Input: part model. Units: mm. Frame: model coordinates. A direction names the side the tool comes from. Give positions to 0.01 mm unless a question says otherwise; leave off trailing zeros. Loops run counter-clockwise (first coordinate to the right, second up) from the corner with the lowest first, then second, coordinate; pieces in that order, holes last. Notation, with made-up numbers: (-12.5, 3) -> (3.5, 3) arc R18 cw to (3.5, 25) -> close; hole circle Ø3 at (86, 36). An arc over 180 degrees is marked (long way). Answer in a Markdown table with one row per item. Add a question column.
```python
from build123d import *

# Parameters (mm, degrees)
SKETCH_2_R               = 101.541015805
CUT_EXTRUDE_1_DEPTH      = 92
SKETCH_4_R               = 60
SKETCH_4_R_2             = 39
EXTRUDE_1_DEPTH          = 1.5
SKETCH_5_W               = 2
SKETCH_5_H               = 2
CUT_EXTRUDE_2_DEPTH      = 94.808315196
CUT_EXTRUDE_2_DEPTH_BACK = 94.808315196
SKETCH_6_OUTSIDE_W       = 156.966
SKETCH_6_OUTSIDE_H       = 156.966
SKETCH_6_OUTSIDE_R       = 52.5
CUT_EXTRUDE_3_DEPTH      = 84.634622017
CUT_EXTRUDE_3_DEPTH_BACK = 84.634622017
SKETCH_7_OUTSIDE_W       = 137.864
SKETCH_7_OUTSIDE_H       = 137.864
SKETCH_7_OUTSIDE_R       = 50.5


with BuildPart() as part:
    # 草图1 → 旋转1 (revolve)
    with BuildSketch(Plane(origin=(0, 0, 0), x_dir=(0, 0, -1), z_dir=(1, 0, 0))):
        with BuildLine():
            Line((-40, 0), (40, 0))
            ThreePointArc((40, 0), (0, 40), (-40, 0))
        make_face()
    revolve(axis=Axis((0, 0, 40), (0, 0, -1)))

    # 草图2 → 切除-拉伸1 (cut)
    with BuildSketch(Plane.XY):
        with Locations((-18.762206379, 13.237665106)):
            Circle(SKETCH_2_R)
    extrude(amount=-CUT_EXTRUDE_1_DEPTH, mode=Mode.SUBTRACT)

    # 草图3 → 切除-旋转1 (revolve, cut)
    with BuildSketch(Plane(origin=(0, 0, 0), x_dir=(1, 0, 0), z_dir=(0, 1, 0))):
        with BuildLine():
            Line((0, 38.5), (0, -38.5))
            ThreePointArc((0, -38.5), (38.5, 0), (0, 38.5))
        make_face()
    revolve(axis=Axis((0, 0, -38.5), (0, 0, 1)), mode=Mode.SUBTRACT)

    # 草图4 → 凸台-拉伸1 (add)
    with BuildSketch(Plane(origin=(0, 0, 0), x_dir=(-1, 0, 0), z_dir=(0, 0, -1))):
        Circle(SKETCH_4_R)
        Circle(SKETCH_4_R_2, mode=Mode.SUBTRACT)
    extrude(amount=-EXTRUDE_1_DEPTH)

    # 草图5 → 旋转2 (revolve)
    with BuildSketch(Plane(origin=(0, 0, 0), x_dir=(1, 0, 0), z_dir=(0, 1, 0)), mode=Mode.PRIVATE) as revolve_2_sk:
        with Locations((-44, 1)):
            Rectangle(SKETCH_5_W, SKETCH_5_H)
    revolve(revolve_2_sk.sketch.rotate(Axis((0, 0, -24.660694069), (0, 0, 1)), 270), axis=Axis((0, 0, -24.660694069), (0, 0, 1)))

    # 草图6 outside → 切除-拉伸2 (cut, two sides: drawn at the far end of the back side and taken through both)
    with BuildSketch(Plane(origin=(0, 0, 0), x_dir=(-1, 0, 0), z_dir=(0, 0, -1)).offset(-CUT_EXTRUDE_2_DEPTH_BACK)):
        Rectangle(SKETCH_6_OUTSIDE_W, SKETCH_6_OUTSIDE_H)
        Circle(SKETCH_6_OUTSIDE_R, mode=Mode.SUBTRACT)
    extrude(amount=CUT_EXTRUDE_2_DEPTH + CUT_EXTRUDE_2_DEPTH_BACK, mode=Mode.SUBTRACT)

    # 草图7 outside → 切除-拉伸3 (cut, two sides: drawn at the far end of the back side and taken through both)
    with BuildSketch(Plane.XY.offset(1.5).offset(-CUT_EXTRUDE_3_DEPTH_BACK)):
        Rectangle(SKETCH_7_OUTSIDE_W, SKETCH_7_OUTSIDE_H)
        Circle(SKETCH_7_OUTSIDE_R, mode=Mode.SUBTRACT)
    extrude(amount=CUT_EXTRUDE_3_DEPTH + CUT_EXTRUDE_3_DEPTH_BACK, mode=Mode.SUBTRACT)


solid = part.part
```
1) Material intervals for line 1 along X through (y, z) = (0, -1.3); line 2 along Z through (x, y) = (-5, 46); line 3 along X through (y, z) = (16, 31.5) (3 decimals), sorted ascending.
2) Pull-direction query (X, two-part tool) for faces 4 (the face through (32, -22, 0)), 5 (the face through (17.235, 41.569, -1.014)), 6 (the face through (36.5, 23.1, -2)); classes: +X half, -X half, draft (parallel to the pull), parting line (faces both ways), or undercut.
3) Pin query (flat end, axial travel): pin 1 (1 mm diameter, centred on x = 38, y = 14.5, fed in from -Z); pin 2 (4 mm diameter, centred on x = -3.5, z = 22, fed in from +Y); pin 3 (1.5 mm diameter, centred on x = 11, y = -19.5, fed in from +Z); pin 4 (1 mm diameter, centred on x = -35, z = 24, fed in from -Y). Return the tip coordinate at first contact, or that it passes through.
4) Section C-C on z = 13. Output: boundary loops of the cut face in (x, y), and give its area (3 significant figures).
5) Reachability of faces 1 (the face through (-29.061, -31.693, -1.014)), 2 (the face through (-37.2, 15.2, 1.5)), 3 (the face through (-10.95, -49.3, 0.74)) from +Z, -Z, +X, -X, +Y, -Y: full face, straight path, thin tool, end or side. Return the list, or none.
6) Section B-B on y = 0. Output: boundary loops of the cut face in (x, z).
Working result:
| question | item | result |
|---|---|---|
| 1 | line 1 | x = -45 to -43, 43 to 45 |
| 1 | line 2 | z = 0 to 1.5 |
| 1 | line 3 | x = -18.755 to -15.297, 15.297 to 18.755 |
| 2 | face 4 | undercut |
| 2 | face 5 | parting line |
| 2 | face 6 | draft |
| 3 | pin 1 | stops at z = 0 |
| 3 | pin 2 | stops at y = 34.48 |
| 3 | pin 3 | stops at z = 33.64 |
| 3 | pin 4 | passes through |
| 4 | outline | circle Ø75.66 at (0, 0); hole circle Ø72.48 at (0, 0) |
| 4 | area | 370 mm2 |
| 5 | face 1 | -Z |
| 5 | face 2 | +Z |
| 5 | face 3 | +Z, -Z |
| 6 | outline | (-50.5, 0) -> (-45, 0) -> (-45, -2) -> (-43, -2) -> (-43, 0) -> (-38.5, 0) arc R38.5 cw to (38.5, 0) -> (43, 0) -> (43, -2) -> (45, -2) -> (45, 0) -> (50.5, 0) -> (50.5, 1.5) -> (39.97, 1.5) arc R40 ccw to (-39.97, 1.5) -> (-50.5, 1.5) -> close |
